For this review, use the dimensioned drawing (mm, ordinates from the lowest corner) and the shaded views. Round coordinates to 2 decimals unless told otherwise and drop trailing zeros. Order: outer loops, then holes, each group sorted by start corner. A loop starts at its lowest first (then second) coordinate and runs counter-clockwise, first axis right, second up. Notation, with made-up numbers: M 33,-34.5 L 61,-34.5 A8 cw 61,-20.5 Z; hole C 30,31 d7. An arc over 180 degrees is marked long. Put each result on its own line as item: value.
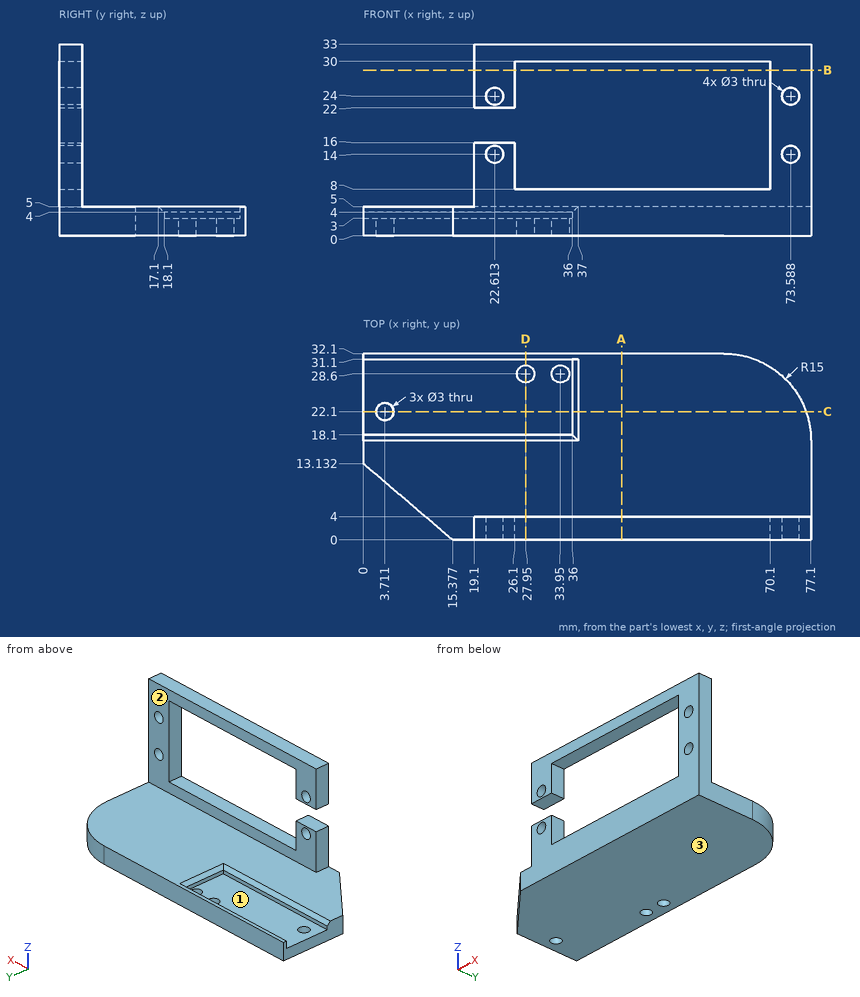
(1) To check wall thickness, follow L1, parallel to X at y = 1.8, z = 14; L2, parallel to Y at x = 33.95, z = 2.15; L3, parallel to Z at x = 24.5, y = 2.5. State the ranges of each line that lie inside material, in increasing order.
A:
L1: x = 19.1 to 21.11, 24.11 to 26.1, 70.1 to 72.09, 75.09 to 77.1
L2: y = 0 to 27.1, 30.1 to 32.1
L3: z = 0 to 16, 22 to 33
(2) Add section B-B on z = 28.5. Give the boundary of the cut face in (x, y).
A:
outline: M 19.1,0 L 26.1,0 L 26.1,4 L 19.1,4 Z; M 70.1,0 L 77.1,0 L 77.1,4 L 70.1,4 Z
(3) Add section A-A on x = 44.5. Give the boundary of the cut face in (y, z).
A:
outline: M 0,0 L 32.1,0 L 32.1,5 L 4,5 L 4,8 L 0,8 Z; M 0,30 L 4,30 L 4,33 L 0,33 Z
(4) Add section C-C on y = 22.1. Give the boundary of the cut face in (x, z), then the cut area to 3 significant figures.
A:
outline: M 0,0 L 2.21,0 L 2.21,3 L 0,3 Z; M 5.21,0 L 76.24,0 L 76.24,5 L 37,5 L 36,4 L 36,3 L 5.21,3 Z
area: 300 mm2
(5) Insertion check: pin 1 Ø4 at (x, y) = (3.711, 22.1) entering from +Z; pin 2 Ø3 at (y, z) = (2.5, 16.5) entering from -X; pin 3 Ø8.5 at (x, z) = (49, 26) entering from +Y. Each pin has a flat end and moves straight along its axis. Give the tip position at first contact, or say it passes through.
A:
pin 1: stops at z = 3
pin 2: stops at x = 19.1
pin 3: stops at y = 4
(6) Add section D-D on x = 27.95. Give the boundary of the cut face in (y, z).
A:
outline: M 0,0 L 27.1,0 L 27.1,3 L 18.1,3 L 18.1,4 L 17.1,5 L 4,5 L 4,8 L 0,8 Z; M 0,30 L 4,30 L 4,33 L 0,33 Z; M 30.1,0 L 32.1,0 L 32.1,5 L 31.1,5 L 31.1,3 L 30.1,3 Z
(7) Draft analysis for pull direction Y (two halves, no side actions). For the marked faces 1, 2 and 3, state which applies: released by +Y, released by -Y, zero draft, split by the parting line, or undercut.
A:
face 1: undercut
face 2: released by +Y
face 3: zero draft
